Design review of the part built by this model. Coordinates are the model's own, in mm. Round coordinates to 2 decimals unless told otherwise and drop trailing zeros. Loops run counter-clockwise (first coordinate to the right, second up) from the corner with the lowest first, then second, coordinate; pieces in that order, holes last. Notation, with made-up numbers: (70.25, -21.75) - (120.25, -21.75) arc R16 ccw to (120.25, -10.75) - close; hole circle Ø11 at (-24, 30.5). An arc over 180 degrees is marked (long way). Return JSON: item names as keys, results as strings. Group by question number.
(1) We need section C-C, the plane x = 0. Write out the cut boundary in (y, z), and give its area (3 significant figures).
(2) We need section A-A, the plane z = -178.5. Write out the cut boundary in (x, y), and give its area (3 significant figures).
(3) Wall thickness on L1, parallel to Z at x = 0, y = 9.2; L2, parallel to Y at x = 6.5, z = 193.5; L3, parallel to X at y = -4.75, z = -61.5: over which ranges is each line inside the solid? List them lowest first. Write a range as [from, to].
(4) We need section D-D, the plane z = 295. Write out the cut boundary in (x, y).
(5) Clearance check with flat-ended pins moving along their axes: pin 1 (6.5 mm diameter, centred on x = 0, z = -255, fed in from +Y); pin 2 (2 mm diameter, centred on x = -2, y = -5.5, fed in from +Z). State where each tip first meets the part, or that it passes through.
(6) We need section B-B, the plane y = 4.5. Write out the cut boundary in (x, z), and give its area (3 significant figures).
Autodesk Inventor part; units mm, degrees
ref_plane "YZ Plane" through (0, 0, 0) normal (1, 0, 0) x (0, 1, 0)
ref_plane "XZ Plane" through (0, 0, 0) normal (0, 1, 0) x (-1, 0, 0)
ref_plane "XY Plane" through (0, 0, 0) normal (0, 0, 1) x (1, 0, 0)
sketch "Sketch1" plane through (0, 0, 0) normal (0, 0, 1) x (1, 0, 0)
  line L0 (-20, 10) -> (20, 10)
  line L1 (20, 10) -> (20, -10)
  line L2 (20, -10) -> (-20, -10)
  line L3 (-20, -10) -> (-20, 10)
  line L4 (-20, 10) -> (20, -10) construction
  line L5 (20, 10) -> (-20, -10) construction
  line L6 (18, 8) -> (-18, 8)
  line L7 (-18, 8) -> (-18, -8)
  line L8 (-18, -8) -> (18, -8)
  line L9 (18, -8) -> (18, 8)
  point P0 (0, 0)
  dimension "d0" = 40
  dimension "d1" = 20
  dimension "d2" = 2
extrude "Extrusion1" add sketch "Sketch1" along normal mid plane 620
fillet "Fillet1" radius 2 4 edges at (-20, 10, 0) (-20, -10, 0) (20, -10, 0) (20, 10, 0)
sketch "Sketch4" plane through (0, 0, 0) normal (0, 1, 0) x (-1, 0, 0)
  circle A0 centre (0, 255) radius 5.5
  line L0 (46.2729, 0) -> (-46.2729, 0) construction
  line L1 (-18, 310) -> (18, 310)
  circle A1 centre (0, 295) radius 5.5
  point P0 (0, 0)
  point P1 (0, 0)
  point P2 (0, 310)
  dimension "d20" = 11
  dimension "d21" = 55
  dimension "d24" = 40
extrude "Extrusion4" cut sketch "Sketch4" along normal through all
mirror "Mirror3" about plane through (0, 0, 0) normal (0, 0, 1) of "Extrusion4"
properties part number "Short tube 3"
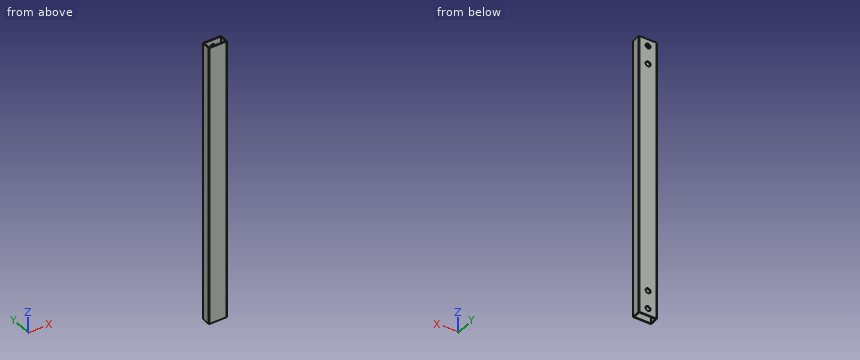
Solutions:
{
 "1": {"outline": "(-10, -310) - (-8, -310) - (-8, 310) - (-10, 310) - close; (8, -310) - (10, -310) - (10, -300.5) - (8, -300.5) - close; (8, -289.5) - (10, -289.5) - (10, -260.5) - (8, -260.5) - close; (8, -249.5) - (10, -249.5) - (10, 249.5) - (8, 249.5) - close; (8, 260.5) - (10, 260.5) - (10, 289.5) - (8, 289.5) - close; (8, 300.5) - (10, 300.5) - (10, 310) - (8, 310) - close", "area": "2,390 mm^2"},
 "2": {"outline": "(-20, -8) arc R2 ccw to (-18, -10) - (18, -10) arc R2 ccw to (20, -8) - (20, 8) arc R2 ccw to (18, 10) - (-18, 10) arc R2 ccw to (-20, 8) - close; hole (-18, -8) - (18, -8) - (18, 8) - (-18, 8) - close", "area": "221 mm^2"},
 "3": {"L1": "[-310, -300.5], [-289.5, -260.5], [-249.5, 249.5], [260.5, 289.5], [300.5, 310]", "L2": "[-10, -8], [8, 10]", "L3": "[-20, -18], [18, 20]"},
 "4": {"outline": "(-20, -8) arc R2 ccw to (-18, -10) - (18, -10) arc R2 ccw to (20, -8) - (20, 8) arc R2 ccw to (18, 10) - (5.5, 10) - (5.5, 8) - (18, 8) - (18, -8) - (-18, -8) - (-18, 8) - (-5.5, 8) - (-5.5, 10) - (-18, 10) arc R2 ccw to (-20, 8) - close"},
 "5": {"pin 1": "y = -8", "pin 2": "through"},
 "6": {"outline": "(-20, -310) - (-18, -310) - (-18, 310) - (-20, 310) - close; (18, -310) - (20, -310) - (20, 310) - (18, 310) - close", "area": "2,480 mm^2"}
}
